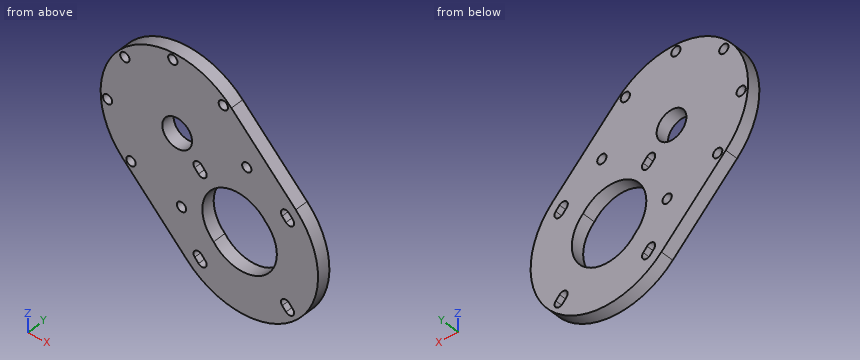
```python
from build123d import *

# Parameters (mm, degrees)
SKETCH2_R           = 8
BOSS_EXTRUDE1_DEPTH = 7
SKETCH6_R           = 2.5
CUT_EXTRUDE2_DEPTH  = 10
CIRPATTERN1_COUNT   = 8


with BuildPart() as part:
    # Sketch2 → Boss-Extrude1 (new body)
    with BuildSketch(Plane(origin=(0, 0, 0), x_dir=(1, 0, 0), z_dir=(0, 1, 0))):
        with BuildLine():
            Line((57.48567214, -39.461643712), (92.069504062, -4.710791287))
            ThreePointArc((92.069504062, -4.710791287), (91.929351462, 53.470307056), (33.748253119, 53.330154455))
            Line((33.748253119, 53.330154455), (-0.835578803, 18.579302031))
            ThreePointArc((-0.835578803, 18.579302031), (-0.695426202, -39.601796312), (57.48567214, -39.461643712))
        make_face()
        with Locations(Location((28.325046669, -10.441170841, 0), (0, 0, 270))):
            Circle(SKETCH2_R, mode=Mode.SUBTRACT)
        with BuildLine():
            ThreePointArc((75.857560085, 10.405306461), (75.736496811, 38.325822665), (47.914533773, 35.978855656))
            ThreePointArc((47.914533773, 35.978855656), (48.035597047, 8.058339452), (75.857560085, 10.405306461))
        make_face(mode=Mode.SUBTRACT)
        with BuildLine():
            ThreePointArc((43.521692021, 48.399463186), (43.365065843, 51.936993301), (39.827535728, 51.780367124))
            Line((39.827535728, 51.780367124), (37.781872405, 49.545166072))
            ThreePointArc((37.781872405, 49.545166072), (37.938498583, 46.007635957), (41.476028698, 46.164262134))
            Line((41.476028698, 46.164262134), (43.521692021, 48.399463186))
        make_face(mode=Mode.SUBTRACT)
        with BuildLine():
            ThreePointArc((90.519256192, 48.401692465), (90.362836565, 51.934557472), (86.829971557, 51.778137845))
            Line((86.829971557, 51.778137845), (84.784308234, 49.542936793))
            ThreePointArc((84.784308234, 49.542936793), (84.940727861, 46.010071786), (88.473592869, 46.166491413))
            Line((88.473592869, 46.166491413), (90.519256192, 48.401692465))
        make_face(mode=Mode.SUBTRACT)
        with BuildLine():
            ThreePointArc((43.560284925, 1.364142834), (43.400386196, 4.975586205), (39.788942825, 4.815687476))
            Line((39.788942825, 4.815687476), (37.743279502, 2.580486424))
            ThreePointArc((37.743279502, 2.580486424), (37.903178231, -1.030956947), (41.514621602, -0.871058218))
            Line((41.514621602, -0.871058218), (43.560284925, 1.364142834))
        make_face(mode=Mode.SUBTRACT)
        with BuildLine():
            ThreePointArc((90.568112992, 1.356978562), (90.407550468, 4.983414272), (86.781114757, 4.822851748))
            Line((86.781114757, 4.822851748), (84.735451434, 2.587650696))
            ThreePointArc((84.735451434, 2.587650696), (84.896013958, -1.038785014), (88.522449669, -0.87822249))
            Line((88.522449669, -0.87822249), (90.568112992, 1.356978562))
        make_face(mode=Mode.SUBTRACT)
    extrude(amount=BOSS_EXTRUDE1_DEPTH)

    # Sketch6 → Cut-Extrude2 (cut)
    with BuildSketch(Plane(origin=(0, 7, 0), x_dir=(1, 0, 0), z_dir=(0, 1, 0))):
        with Locations(Location((3.517083482, 17.6802616, 0), (0, 0, 270))):
            Circle(SKETCH6_R)
    cut_extrude2 = extrude(amount=-CUT_EXTRUDE2_DEPTH, mode=Mode.SUBTRACT)

    # CirPattern1: Cut-Extrude2 ×8 about axis
    cirpattern1_axis = Axis((28.325046669, 0, 10.441170841), (0, 1, 0))
    for i in range(1, CIRPATTERN1_COUNT):
        add(cut_extrude2.rotate(cirpattern1_axis, i * 360 / CIRPATTERN1_COUNT), mode=Mode.SUBTRACT)


solid = part.part
```
The listing builds one solid part. Answer for the finished solid, in the listing's coordinates (mm). Round coordinates to 2 decimals unless told otherwise and drop trailing zeros. Loops run counter-clockwise (first coordinate to the right, second up) from the corner with the lowest first, then second, coordinate; pieces in that order, holes last.
1) A cutting plane is placed at C-C on x = 25. Determine the outline of the cut face in (y, z).
Outcome:
outline: (0, -44.54) - (7, -44.54) - (7, 3.16) - (0, 3.16) - close; (0, 17.72) - (7, 17.72) - (7, 45.57) - (0, 45.57) - close; (0, 50.17) - (7, 50.17) - (7, 51.45) - (0, 51.45) - close
2) Given P1, Ø4, axis at x = 30.67, z = -26.99, coming from the -Y side; P2, Ø6.5, axis at x = 25.98, z = 47.87, coming from the +Y side; P3, Ø2, axis at y = 5.5, z = 14.5, coming from the +X side, each flat-ended and moving along its own axis, determine where each tip first touches the part or whether it passes through.
Outcome:
P1: passes through
P2: stops at y = 7
P3: stops at x = 83.32
3) A cutting plane is placed at B-B on z = -27. Determine the outline of the cut face in (x, y).
Outcome:
outline: (7.54, 0) - (28.17, 0) - (28.17, 7) - (7.54, 7) - close; (33.17, 0) - (42.51, 0) - (42.51, 7) - (33.17, 7) - close; (81.72, 0) - (103.96, 0) - (103.96, 7) - (81.72, 7) - close
4) Consider line 1 (Z direction, x = 84.5, y = 2.75); line 2 (X direction, y = 3.25, z = 11.5); line 3 (Z direction, x = 25, y = 2.5). Determine where each line is inside the solid, lowest interval first.
Outcome:
line 1: z = -59.33 to -49.17, -46.54 to -2.29, 0.58 to 12.32
line 2: x = -12.8 to 20.4, 36.25 to 63.61, 67.9 to 85.31
line 3: z = -44.54 to 3.16, 17.72 to 45.57, 50.17 to 51.45
5) A cutting plane is placed at D-D on y = 2.75. Give the number of separate pieces and of enclosed holes in the cut face, plus the area to 3 significant figures.
Outcome:
separate pieces: 1
enclosed holes: 13
area: 7,620 mm2
6) A cutting plane is placed at A-A on z = -40. Determine the outline of the cut face in (x, y), plus the area to 3 significant figures.
Outcome:
outline: (20.48, 0) - (52.19, 0) - (52.19, 7) - (20.48, 7) - close; (73.62, 0) - (100.94, 0) - (100.94, 7) - (73.62, 7) - close
area: 413 mm2
